For this review, take the finished solid that the model builds, in its own axes (mm). Face numbers are marked on the shaded views. Round coordinates to 2 decimals unless told otherwise and drop trailing zeros. Write each loop counter-clockwise with the first axis right and the second up, starting at its lowest first coordinate (ties: lowest second). Pieces come first, ordered by that corner, then holes. Notation, with made-up numbers: (67.5, -37) - (106.5, -37) arc R14 ccw to (106.5, -19) - close; hole circle Ø4 at (37, -38). An arc over 180 degrees is marked (long way). One line per item, written item: value. Start each with the question number.
Q1. Add section C-C on z = -3. Write out the cut boundary in (x, y).
Q2. Clearance check with flat-ended pins moving along their axes: pin 1 Ø4 at (x, y) = (-0.5, -0.5) entering from +Z; pin 2 Ø5 at (y, z) = (-2, -5.5) entering from -X; pin 3 Ø4 at (x, z) = (2.5, -12) entering from -Y. State where each tip first meets the part, or that it passes through.
Q3. For probe 1 along Y at (x, z) = (0, -16) (3 decimals); probe 2 along Y at (x, z) = (0, -0.15) (3 decimals); probe 3 along Z at (x, y) = (0.5, -1.75), list the stretches that pass through material, from the lowest coordinate up.
Q4. Add section A-A on y = 0. Write out the cut boundary in (x, z) (3 decimals).
Q5. Mouldability with a two-part tool opening along Y and no side actions: class the marked faces 1, 2, 3 and 4 as +Y half, -Y half, draft (parallel to the pull), parting line (faces both ways), or undercut.
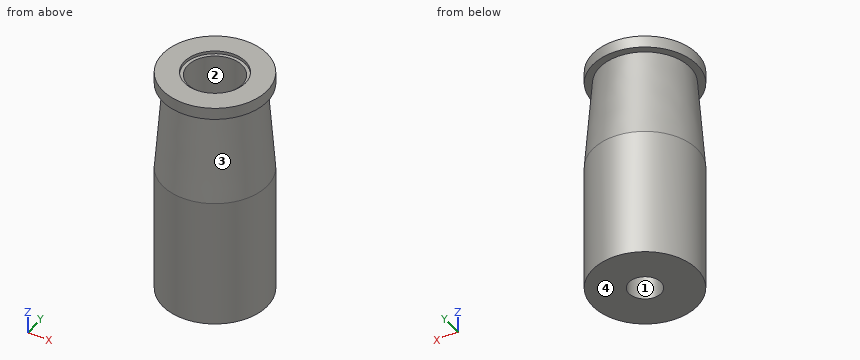
```python
from build123d import *

# Parameters (mm, degrees)
SKETCH2_R          = 2.85
CUT_EXTRUDE1_DEPTH = 0.27
SKETCH3_R          = 2.539141962
CUT_EXTRUDE2_DEPTH = 5
SKETCH4_R          = 1.5
CUT_EXTRUDE3_DEPTH = 19


with BuildPart() as part:
    # Sketch1 → Revolve1 (revolve)
    with BuildSketch(Plane(origin=(0, 0, 0), x_dir=(1, 0, 0), z_dir=(0, 1, 0))):
        Polygon((0, 0), (-4.875, 0), (-4.875, 1.1), (-4.215, 1.1), (-4.875, 9.51), (-4.875, 21.51), (0, 21.51), align=None)
    revolve(axis=Axis((0, 0, -21.51), (0, 0, 1)))

    # Sketch2 → Cut-Extrude1 (cut)
    with BuildSketch(Plane.XY):
        Circle(SKETCH2_R)
    extrude(amount=-CUT_EXTRUDE1_DEPTH, mode=Mode.SUBTRACT)

    # Sketch3 → Cut-Extrude2 (cut)
    with BuildSketch(Plane.XY.offset(-0.27)):
        Circle(SKETCH3_R)
    extrude(amount=-CUT_EXTRUDE2_DEPTH, mode=Mode.SUBTRACT)

    # Sketch4 → Cut-Extrude3 (cut)
    with BuildSketch(Plane(origin=(0, 0, -21.51), x_dir=(-1, 0, 0), z_dir=(0, 0, -1))):
        Circle(SKETCH4_R)
    extrude(amount=-CUT_EXTRUDE3_DEPTH, mode=Mode.SUBTRACT)


solid = part.part
```
Result set:
1. outline: circle Ø8.73 at (0, 0); hole circle Ø5.08 at (0, 0)
2. pin 1: stops at z = -0.27
2. pin 2: stops at x = -4.69
2. pin 3: stops at y = -4.85
3. probe 1: y = -4.875 to -1.5, 1.5 to 4.875
3. probe 2: y = -4.875 to -2.85, 2.85 to 4.875
3. probe 3: z = -21.51 to -5.27
4. outline: (-4.875, -21.51) - (-1.5, -21.51) - (-1.5, -5.27) - (-2.539, -5.27) - (-2.539, -0.27) - (-2.85, -0.27) - (-2.85, 0) - (-4.875, 0) - (-4.875, -1.1) - (-4.215, -1.1) - (-4.875, -9.51) - close; (1.5, -21.51) - (4.875, -21.51) - (4.875, -9.51) - (4.215, -1.1) - (4.875, -1.1) - (4.875, 0) - (2.85, 0) - (2.85, -0.27) - (2.539, -0.27) - (2.539, -5.27) - (1.5, -5.27) - close
5. face 1: undercut
5. face 2: undercut
5. face 3: parting line
5. face 4: draft
